Geometry: final body of the model. Coordinates: model frame, mm. Round coordinates to 2 decimals unless told otherwise and drop trailing zeros. Write each loop counter-clockwise with the first axis right and the second up, starting at its lowest first coordinate (ties: lowest second). Pieces come first, ordered by that corner, then holes. Notation, with made-up numbers: (72, 89.25) - (116, 89.25) arc R21 ccw to (116, 124.25) - close; hole circle Ø10 at (81.5, -28.75). An arc over 180 degrees is marked (long way). Write each question's results on one line, items separated by ' | '.
from build123d import *

# Parameters (mm, degrees)
CROQUIS1_W            = 200
CROQUIS1_H            = 40
EXTRUIR1_DEPTH        = 2.5
REDONDEO1_R           = 10
CROQUIS2_R            = 2.95
CORTAR_EXTRUIR1_DEPTH = 10
CROQUIS3_R            = 2.95
CORTAR_EXTRUIR2_DEPTH = 10
CROQUIS4_R            = 2.95
CORTAR_EXTRUIR3_DEPTH = 10


with BuildPart() as part:
    # Croquis1 → Extruir1 (new, symmetric)
    with BuildSketch(Plane.XY):
        with Locations((-25, -5)):
            Rectangle(CROQUIS1_W, CROQUIS1_H)
    extrude(amount=EXTRUIR1_DEPTH, both=True)

    # Redondeo1
    redondeo1_edges = [part.edges().sort_by_distance(p)[0] for p in [
        (75, 15, 0),
        (75, -25, 0),
        (-125, -25, 0),
        (-125, 15, 0),
    ]]
    fillet(redondeo1_edges, radius=REDONDEO1_R)

    # Croquis2 → Cortar-Extruir1 (cut)
    with BuildSketch(Plane(origin=(0, 0, -2.5), x_dir=(-1, 0, 0), z_dir=(0, 0, -1))):
        with Locations((73.999510292, -4.90303525)):
            Circle(CROQUIS2_R)
    extrude(amount=-CORTAR_EXTRUIR1_DEPTH, mode=Mode.SUBTRACT)

    # Croquis3 → Cortar-Extruir2 (cut)
    with BuildSketch(Plane.XY.offset(2.5)):
        with Locations((-45, 5)):
            Circle(CROQUIS3_R)
        with Locations((-5, 5)):
            Circle(CROQUIS3_R)
        with Locations((-45, -15)):
            Circle(CROQUIS3_R)
        with Locations((-5, -15)):
            Circle(CROQUIS3_R)
    extrude(amount=-CORTAR_EXTRUIR2_DEPTH, mode=Mode.SUBTRACT)

    # Croquis4 → Cortar-Extruir3 (cut)
    with BuildSketch(Plane.XY.offset(2.5)):
        with Locations((45.400489708, -4.90303525)):
            Circle(CROQUIS4_R)
    extrude(amount=-CORTAR_EXTRUIR3_DEPTH, mode=Mode.SUBTRACT)


solid = part.part
Q1. Section query B-B, the plane z = -1.05. Return loops of the section in (x, y), plus the area to 3 significant figures.
Answer block:
outline: (-125, -15) arc R10 ccw to (-115, -25) - (65, -25) arc R10 ccw to (75, -15) - (75, 5) arc R10 ccw to (65, 15) - (-115, 15) arc R10 ccw to (-125, 5) - close; hole circle Ø5.9 at (-74, -4.9); hole circle Ø5.9 at (-45, -15); hole circle Ø5.9 at (-45, 5); hole circle Ø5.9 at (-5, -15); hole circle Ø5.9 at (-5, 5); hole circle Ø5.9 at (45.4, -4.9) | area: 7,750 mm2
Q2. Mould query, pull axis Y, two halves, no side actions, for faces 1 (the cylindrical face through (-122.15, -21.99, 0.04)), 2 (the cylindrical face through (-122.15, 11.99, -0.04)), 3 (the cylindrical face through (-76.813, -4.017, -0.035)), 4 (the flat face through (75, -5, 0)). Classes: pulls with the +Y half, pulls with the -Y half, needs draft (parallel to the pull), parting line crosses it, or undercut.
Answer block:
face 1: pulls with the -Y half | face 2: pulls with the +Y half | face 3: undercut | face 4: needs draft
Q3. Ray query, line 1 along Y through (x, z) = (-45, -0.7); line 2 along X through (y, z) = (-6, -0.7); line 3 along Y through (x, z) = (-4, -1.4). Return the intervals inside material, ascending.
Answer block:
line 1: -25 to -17.95, -12.05 to 2.05, 7.95 to 15 | line 2: -125 to -76.74, -71.26 to 42.66, 48.14 to 75 | line 3: -25 to -17.78, -12.22 to 2.22, 7.78 to 15
Q4. Section query A-A, the plane x = -5. Return loops of the section in (y, z), plus the area to 3 significant figures.
Answer block:
outline: (-25, -2.5) - (-17.95, -2.5) - (-17.95, 2.5) - (-25, 2.5) - close; (-12.05, -2.5) - (2.05, -2.5) - (2.05, 2.5) - (-12.05, 2.5) - close; (7.95, -2.5) - (15, -2.5) - (15, 2.5) - (7.95, 2.5) - close | area: 141 mm2
Q5. Pin query (flat end, axial travel): pin 1 (4.5 mm diameter, centred on x = -74, y = -4.9, fed in from +Z). Return the tip coordinate at first contact, or that it passes through.
Answer block:
pin 1: through
